Here's the drawing with two shaded views (mm, measured from the low corner). I have some questions. A direction names the side the tool comes from. Round coordinates to 2 decimals unless told otherwise and drop trailing zeros. Order: outer loops, then holes, each group sorted by start corner. A loop starts at its lowest first (then second) coordinate and runs counter-clockwise, first axis right, second up. Notation, with made-up numbers: (24.25, -18) - (56.25, -18) arc R29 cw to (56.25, 4) - close; hole circle Ø11 at (30.25, 29). An arc over 180 degrees is marked (long way). Return JSON: item names as keys, results as strings. Group by question number.
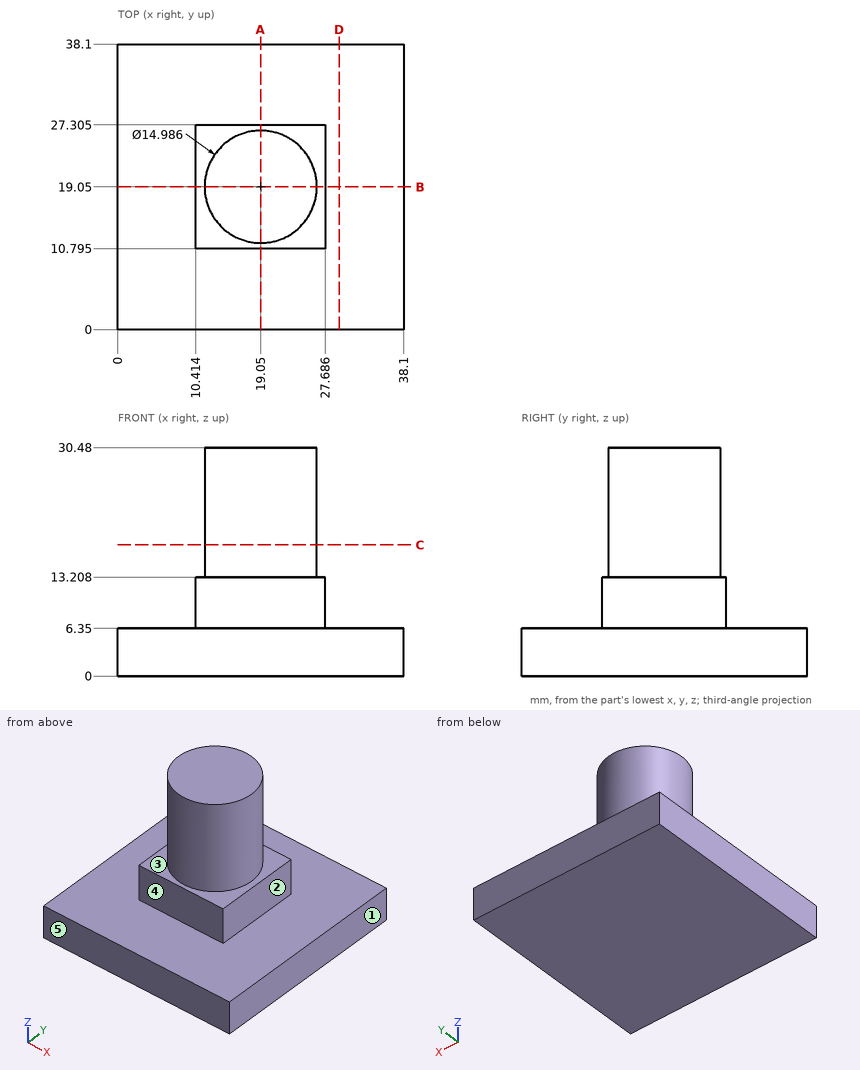
1) If I drill on line 1 along Z through (x, y) = (8, 4); line 2 along Y through (x, z) = (19, 14.5); line 3 along Z through (x, y) = (26, 22), over which ranges is the centre line in solid material (lowest first)? Write a range as from..to.
2) I want a section at B-B, the plane y = 19.05. List the corners of the cut face in (x, z) for me, plus the area to 3 significant figures.
3) For the marked faces 1, 2, 3, 4 and 5, which set-ups out of +Z, -Z, +X, -X, +Y, -Y let a thin tool reach every point of the face, with its end or its side?
4) I want a section at D-D, the plane x = 29.5. List the corners of the cut face in (y, z) for me.
5) Will these pins go through, and if not, where does the flat tip stop? pin 1 (7.5 mm diameter, centred on y = 16.5, z = 10, fed in from +X); pin 2 (12 mm diameter, centred on x = 29, y = 34.5, fed in from +Z); pin 3 (6 mm diameter, centred on x = 14, z = 21, fed in from +Y); pin 4 (1 mm diameter, centred on x = 17.5, z = 23, fed in from +Y).
6) I want a section at C-C, the plane z = 17.5. List the corners of the cut face in (x, y) for me, plus the area to 3 significant figures.
7) I want a section at A-A, the plane x = 19.05. List the corners of the cut face in (y, z) for me (3 decimals), plus the area to 3 significant figures.
Outcome:
{
 "1": {"line 1": "0..6.35", "line 2": "11.56..26.54", "line 3": "0..13.21"},
 "2": {"outline": "(0, 0) - (38.1, 0) - (38.1, 6.35) - (27.69, 6.35) - (27.69, 13.21) - (26.54, 13.21) - (26.54, 30.48) - (11.56, 30.48) - (11.56, 13.21) - (10.41, 13.21) - (10.41, 6.35) - (0, 6.35) - close", "area": "619 mm^2"},
 "3": {"face 1": "+Z, -Z, +X, +Y, -Y", "face 2": "+Z, +X, +Y, -Y", "face 3": "+Z", "face 4": "+Z, +X, -X, -Y", "face 5": "+Z, -Z, +X, -X, -Y"},
 "4": {"outline": "(0, 0) - (38.1, 0) - (38.1, 6.35) - (0, 6.35) - close"},
 "5": {"pin 1": "x = 38.1", "pin 2": "z = 6.35", "pin 3": "y = 26.26", "pin 4": "y = 26.47"},
 "6": {"outline": "circle Ø14.99 at (19.05, 19.05)", "area": "176 mm^2"},
 "7": {"outline": "(0, 0) - (38.1, 0) - (38.1, 6.35) - (27.305, 6.35) - (27.305, 13.208) - (26.543, 13.208) - (26.543, 30.48) - (11.557, 30.48) - (11.557, 13.208) - (10.795, 13.208) - (10.795, 6.35) - (0, 6.35) - close", "area": "614 mm^2"}
}
